For this review, use the dimensioned drawing (mm, ordinates from the lowest corner) and the shaded views. Give positions to 0.01 mm unless a question says otherwise; leave off trailing zeros. Loops run counter-clockwise (first coordinate to the right, second up) from the corner with the lowest first, then second, coordinate; pieces in that order, holes last. Notation, with made-up numbers: M -4,87.5 L 24,87.5 A22 ccw 24,115.5 Z; hole C -27,63 d2. An arc over 180 degrees is marked long. Return JSON: item names as keys, results as strings.
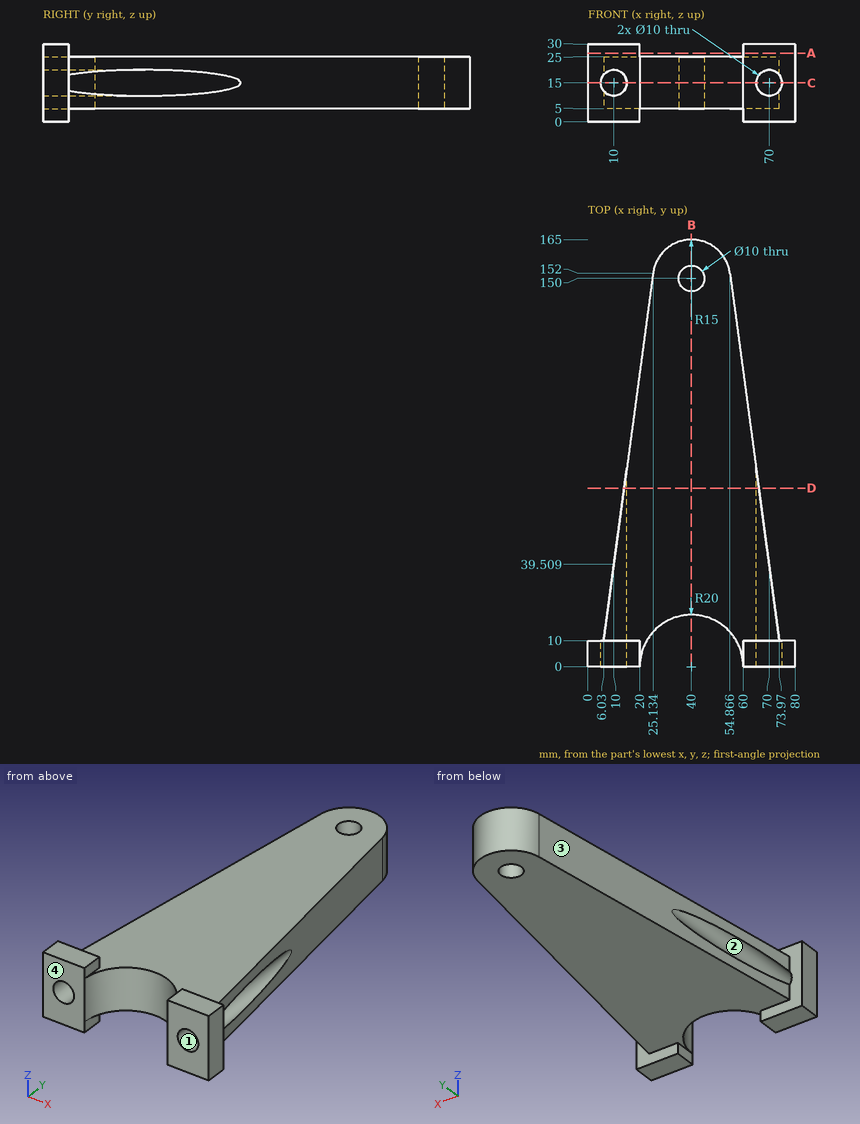
1) Consider section C-C on z = 15. Write out the cut boundary in (x, y), then the cut area to 3 significant figures.
From the geometry:
{"outline": "M 0,0 L 5,0 L 5,10 L 0,10 Z; M 15,0 L 20,0 A20 cw 60,0 L 65,0 L 65,76.67 L 54.87,152 A15 ccw 25.13,152 L 15,76.67 Z; M 75,0 L 80,0 L 80,10 L 75,10 Z; hole C 40,150 d10", "area": "6,520 mm²"}
2) Consider section D-D on y = 69. Write out the cut boundary in (x, z), then the cut area to 3 significant figures.
From the geometry:
{"outline": "M 13.97,5 L 66.03,5 L 66.03,11.96 A5 cw 66.03,18.04 L 66.03,25 L 13.97,25 L 13.97,18.04 A5 cw 13.97,11.96 Z", "area": "1,030 mm²"}
3) Consider section A-A on z = 26.5. Write out the cut boundary in (x, y).
From the geometry:
{"outline": "M 0,0 L 20,0 L 20,10 L 0,10 Z; M 60,0 L 80,0 L 80,10 L 60,10 Z"}
4) Insertion check: pin 1 (10 mm diameter, centred on x = 53.5, y = 92.5, fed in from +Z); pin 2 (10 mm diameter, centred on y = 55.5, z = 22, fed in from +X); pin 3 (3 mm diameter, centred on x = 21, y = 130, fed in from -Z); pin 4 (8 mm diameter, centred on x = 70, z = 15, fed in from +Y). Each pin has a flat end and moves straight along its axis. Give the tip position at first contact, or say it passes through.
From the geometry:
{"pin 1": "z = 25", "pin 2": "x = 68.52", "pin 3": "z = 5", "pin 4": "through"}
5) Wall thickness on L1, parallel to Z at x = 70, y = 20; L2, parallel to Z at x = 54, y = 145.5; L3, parallel to Y at x = 43, z = 21.5: over which ranges is each line inside the solid? List them lowest first. Write a range as from..to.
From the geometry:
{"L1": "5..10, 20..25", "L2": "5..25", "L3": "19.77..146, 154..164.7"}
6) The part is to be moulded in two halves that separate along X. For the marked faces 1, 2, 3 and 4, say which applies: released by +X, released by -X, zero draft, split by the parting line, or undercut.
From the geometry:
{"face 1": "undercut", "face 2": "undercut", "face 3": "released by -X", "face 4": "zero draft"}
7) Consider section B-B on x = 40. Write out the cut boundary in (y, z).
From the geometry:
{"outline": "M 20,5 L 145,5 L 145,25 L 20,25 Z; M 155,5 L 165,5 L 165,25 L 155,25 Z"}
